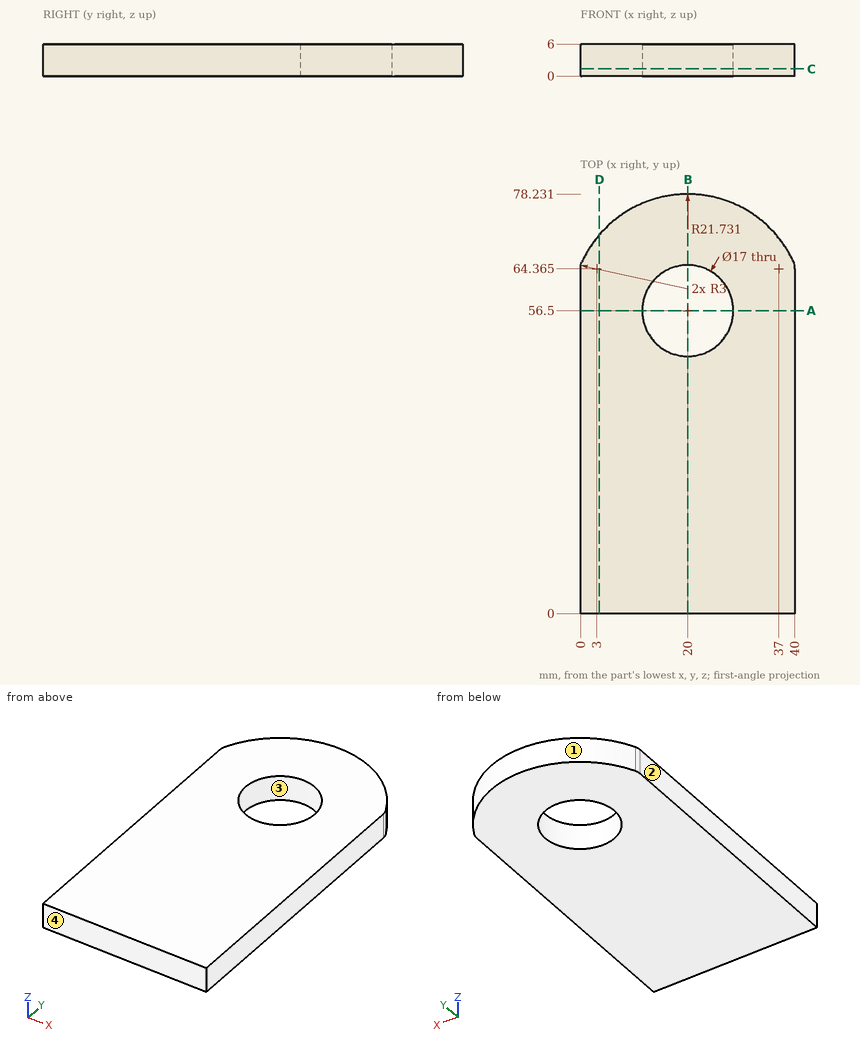
The drawing under review shows one solid part. Ordinate dimensions are in mm from its lowest x, y, z. Round coordinates to 2 decimals unless told otherwise and drop trailing zeros. Order: outer loops, then holes, each group sorted by start corner. A loop starts at its lowest first (then second) coordinate and runs counter-clockwise, first axis right, second up. Notation, with made-up numbers: (40, 33) - (68, 33) arc R27 ccw to (68, 60) - close; hole circle Ø4 at (32, 39). An arc over 180 degrees is marked (long way). Return JSON: item names as keys, results as strings.
Q1. Consider section B-B on x = 20. Write out the cut boundary in (y, z), plus the area to 3 significant figures.
Computed values:
{"outline": "(0, 0) - (48, 0) - (48, 6) - (0, 6) - close; (65, 0) - (78.23, 0) - (78.23, 6) - (65, 6) - close", "area": "367 mm2"}
Q2. The part is to be moulded in two halves that separate along Y. For the marked faces 1, 2, 3 and 4, say which applies: pulls with the +Y half, pulls with the -Y half, needs draft (parallel to the pull), parting line crosses it, or undercut.
Computed values:
{"face 1": "pulls with the +Y half", "face 2": "needs draft", "face 3": "undercut", "face 4": "pulls with the -Y half"}
Q3. Wall thickness on L1, parallel to Y at x = 20, z = 4.3; L2, parallel to X at y = 54, z = 3.3 (1 decimal); L3, parallel to Y at x = 14, z = 5.65 (1 decimal): over which ranges is each line inside the solid? List them lowest first. Write a range as [from, to].
Computed values:
{"L1": "y = [0, 48], [65, 78.23]", "L2": "x = [0, 11.9], [28.1, 40]", "L3": "y = [0, 50.5], [62.5, 77.4]"}
Q4. Consider section D-D on x = 3.5. Write out the cut boundary in (y, z).
Computed values:
{"outline": "(0, 0) - (70.64, 0) - (70.64, 6) - (0, 6) - close"}
Q5. For pin 1 Ø10 at (x, y) = (11, 42) entering from -Z; pin 2 Ø10 at (x, y) = (20, 56.5) entering from +Z; pin 3 Ø2 at (y, z) = (66.5, 5) entering from +X, all flat-tipped, find the tip position at first contact; note any pin that passes through.
Computed values:
{"pin 1": "stops at z = 0", "pin 2": "passes through", "pin 3": "stops at x = 39.78"}
Q6. Consider section C-C on z = 1.35. Write out the cut boundary in (x, y) (1 decimal), plus the area to 4 significant figures.
Computed values:
{"outline": "(0, 0) - (40, 0) - (40, 64.4) arc R3 ccw to (39.7, 65.6) arc R21.7 ccw to (0.3, 65.6) arc R3 ccw to (0, 64.4) - close; hole circle Ø17 at (20, 56.5)", "area": "2,755 mm2"}
Q7. Consider section A-A on y = 56.5. Write out the cut boundary in (x, z), plus the area to 3 significant figures.
Computed values:
{"outline": "(0, 0) - (11.5, 0) - (11.5, 6) - (0, 6) - close; (28.5, 0) - (40, 0) - (40, 6) - (28.5, 6) - close", "area": "138 mm2"}
